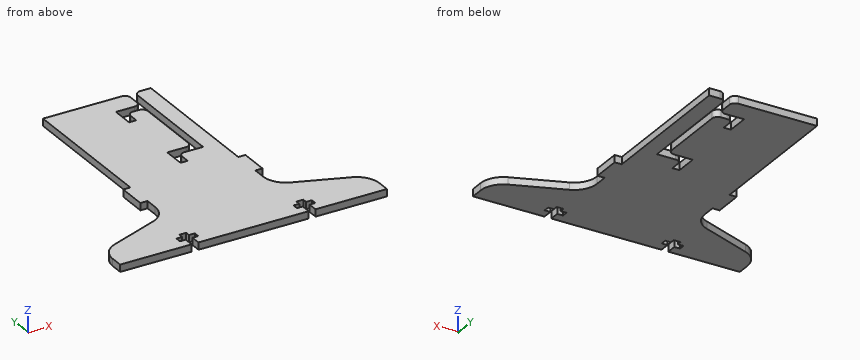
from build123d import *

# Parameters (mm, degrees)
BOSS_EXTRUDE1_DEPTH = 3.175
SKETCH2_W           = 5.42671
SKETCH2_H           = 83.83778
SKETCH2_W_2         = 23.424388
BOSS_EXTRUDE2_DEPTH = 3.175
SKETCH3_W           = 3.175
SKETCH3_H           = 64.78778
SKETCH3_H_2         = 6.35
CUT_EXTRUDE2_DEPTH  = 92.344542194
BOSS_EXTRUDE4_DEPTH = 3.175
FILLET1_R           = 10.16
CUT_EXTRUDE5_DEPTH  = 109.16364837
FILLET2_R           = 2.54


with BuildPart() as part:
    # Sketch1 → Boss-Extrude1 (new body)
    with BuildSketch(Plane.XY):
        Polygon((4.470127528, 71.013782114), (4.470127528, 36.088782114), (-6.35, 36.088782114), (-6.35, 32.913782114), (-6.35, 26.309782114), (-3.175, 26.309782114), (-3.175, 32.913782114), (7.645127528, 32.913782114), (7.645127528, 83.83778), (12.7, 83.83778), (12.7, 0), (-12.7, 0), (-12.7, 83.83778), (4.470127528, 83.83778), (4.470127528, 74.188782114), (-6.35, 74.188782114), (-6.35, 71.013782114), (-6.35, 64.409782114), (-3.175, 64.409782114), (-3.175, 71.013782114), align=None)
    extrude(amount=BOSS_EXTRUDE1_DEPTH)

    # Sketch2 → Boss-Extrude2 (add)
    with BuildSketch(Plane.XY):
        with Locations((15.413355, 41.91889)):
            Rectangle(SKETCH2_W, SKETCH2_H)
        with Locations((-24.412194, 41.91889)):
            Rectangle(SKETCH2_W_2, SKETCH2_H)
    extrude(amount=BOSS_EXTRUDE2_DEPTH)

    # Sketch3 → Cut-Extrude2 (cut, through all)
    with BuildSketch(Plane.XY):
        with Locations((-34.536888, 51.44389)):
            Rectangle(SKETCH3_W, SKETCH3_H)
        with Locations((16.53921, 51.44389)):
            Rectangle(SKETCH3_W, SKETCH3_H)
        with Locations((-34.536888, 3.175)):
            Rectangle(SKETCH3_W, SKETCH3_H_2)
        with Locations((16.53921, 3.175)):
            Rectangle(SKETCH3_W, SKETCH3_H_2)
    extrude(amount=CUT_EXTRUDE2_DEPTH, mode=Mode.SUBTRACT)

    # Sketch5 → Boss-Extrude4 (add)
    with BuildSketch(Plane.XY):
        Polygon((-32.949388, 0), (-32.949388, -6.35), (-68.268007503, -19.717143922), (-68.268007503, -32.282068045), (50.270329503, -32.282068045), (50.270329503, -19.717143922), (14.95171, -6.35), (14.95171, 0), align=None)
    extrude(amount=BOSS_EXTRUDE4_DEPTH)

    # Fillet1
    fillet1_edges = [part.edges().sort_by_distance(p)[0] for p in [
        (-32.949388, -6.35, 1.5875),
        (-68.268007503, -19.717143922, 1.5875),
        (50.270329503, -19.717143922, 1.5875),
        (14.95171, -6.35, 1.5875),
    ]]
    fillet(fillet1_edges, radius=FILLET1_R)

    # Sketch6 → Cut-Extrude5 (cut, through all)
    with BuildSketch(Plane.XY):
        Polygon((-36.518007503, -32.282068045), (-36.518007503, -27.870697677), (-39.076507827, -27.870697677), (-39.076507827, -25.312197354), (-36.518007503, -25.312197354), (-36.518007503, -23.233415841), (-33.479788369, -23.233415841), (-33.479788369, -25.312197354), (-30.921288046, -25.312197354), (-30.921288046, -27.870697677), (-33.479788369, -27.870697677), (-33.479788369, -32.282068045), align=None)
        Polygon((15.482110369, -32.282068045), (15.482110369, -27.870697677), (12.923610046, -27.870697677), (12.923610046, -25.312197354), (15.482110369, -25.312197354), (15.482110369, -23.233415841), (18.520329503, -23.233415841), (18.520329503, -25.312197354), (21.078829827, -25.312197354), (21.078829827, -27.870697677), (18.520329503, -27.870697677), (18.520329503, -32.282068045), align=None)
    extrude(amount=CUT_EXTRUDE5_DEPTH, mode=Mode.SUBTRACT)

    # Fillet2
    fillet2_edges = [part.edges().sort_by_distance(p)[0] for p in [
        (4.470127528, 83.83778, 1.5875),
        (4.470127528, 74.188782114, 1.5875),
        (-3.175, 71.013782114, 1.5875),
        (4.470127528, 71.013782114, 1.5875),
        (4.470127528, 36.088782114, 1.5875),
        (-3.175, 32.913782114, 1.5875),
        (7.645127528, 83.83778, 1.5875),
    ]]
    fillet(fillet2_edges, radius=FILLET2_R)


solid = part.part
Read the model definition and answer for the solid it produces. Units are mm, in the model's axes. Coordinates: 2 decimals unless noted, no trailing zeros. Order: outer loops, then holes, each group sorted by start corner. A loop starts at its lowest first (then second) coordinate and runs counter-clockwise, first axis right, second up. Notation, with made-up numbers: (81.25, 24) - (107.25, 24) arc R16 ccw to (107.25, 39) - close; hole circle Ø3 at (89, -0.75). An arc over 180 degrees is marked (long way). Use one line per item in the form item = value.
(1) Straight lines are drawn through the part: L1, parallel to X at y = 65, z = 2.9 (3 decimals); L2, parallel to X at y = -27, z = 1.35; L3, parallel to X at y = 39, z = 1.4. For each, find the intervals that lie inside material, in ascending order.
Computed values:
L1 = -32.949 to -6.35, -3.175 to 4.47, 7.645 to 14.952
L2 = -68.27 to -39.08, -30.92 to 12.92, 21.08 to 50.27
L3 = -32.95 to 4.47, 7.65 to 14.95
(2) Section A-A, the plane y = 42 is taken. Give the vertices of the cut face in (x, z) (3 decimals), then the cut area to 3 significant figures.
Computed values:
outline = (-32.949, 0) - (4.47, 0) - (4.47, 3.175) - (-32.949, 3.175) - close; (7.645, 0) - (14.952, 0) - (14.952, 3.175) - (7.645, 3.175) - close
area = 142 mm²
(3) Given pin 1 Ø0.9 at (x, z) = (17, 1.5) entering from -Y; pin 2 Ø1 at (y, z) = (3.5, 2.5) entering from +X, each flat-ended and moving along its own axis, determine where each tip first touches the part or whether it passes through.
Computed values:
pin_1 = -23.23
pin_2 = 14.95
(4) Section B-B, the plane x = -51 is taken. Give the vertices of the cut face in (y, z) (3 decimals), then the cut area to 3 significant figures.
Computed values:
outline = (-32.282, 0) - (-13.182, 0) - (-13.182, 3.175) - (-32.282, 3.175) - close
area = 60.6 mm²
